Read the model definition and answer for the solid it produces. Units are mm, in the model's axes. Round coordinates to 2 decimals unless told otherwise and drop trailing zeros. Order: outer loops, then holes, each group sorted by start corner. A loop starts at its lowest first (then second) coordinate and runs counter-clockwise, first axis right, second up.
from build123d import *

# Parameters (mm, degrees)
BOSS_EXTRUDE1_DEPTH = 2.54
SKETCH2_R           = 2.159
CUT_EXTRUDE1_DEPTH  = 2.54
FILLET1_R           = 5.08
SKETCH3_W           = 2.54
SKETCH3_H           = 6.35
CUT_EXTRUDE4_DEPTH  = 3.54


with BuildPart() as part:
    # Sketch1 → Boss-Extrude1 (new body)
    with BuildSketch(Plane.XY):
        Polygon((35.56, -47.131), (35.56, 17.131), (-35.56, 17.131), (-35.56, -47.131), (-65.56, -47.131), (-65.56, 47.131), (65.56, 47.131), (65.56, -47.131), align=None)
    extrude(amount=BOSS_EXTRUDE1_DEPTH)

    # Sketch2 → Cut-Extrude1 (cut)
    with BuildSketch(Plane.XY.offset(2.54)):
        with Locations((-56.181, 36.4985)):
            Circle(SKETCH2_R)
        with Locations((-56.181, 26.7195)):
            Circle(SKETCH2_R)
        with Locations((-7.921, 36.4985)):
            Circle(SKETCH2_R)
        with Locations((-7.921, 26.7195)):
            Circle(SKETCH2_R)
        Polygon((-11.477, 41.7055), (-52.625, 41.7055), (-52.625, 21.5125), (-11.477, 21.5125), (-11.477, 31.609), align=None)
    extrude(amount=-CUT_EXTRUDE1_DEPTH, mode=Mode.SUBTRACT)

    # Fillet1
    fillet1_edges = [part.edges().sort_by_distance(p)[0] for p in [
        (-65.56, 47.131, 1.27),
        (65.56, 47.131, 1.27),
        (35.56, -47.131, 1.27),
        (-35.56, -47.131, 1.27),
    ]]
    fillet(fillet1_edges, radius=FILLET1_R)

    # Sketch3 → Cut-Extrude4 (cut, through all)
    with BuildSketch(Plane.XY.offset(2.54)):
        with Locations((-52.625, 31.609)):
            Rectangle(SKETCH3_W, SKETCH3_H)
    extrude(amount=-CUT_EXTRUDE4_DEPTH, mode=Mode.SUBTRACT)


solid = part.part
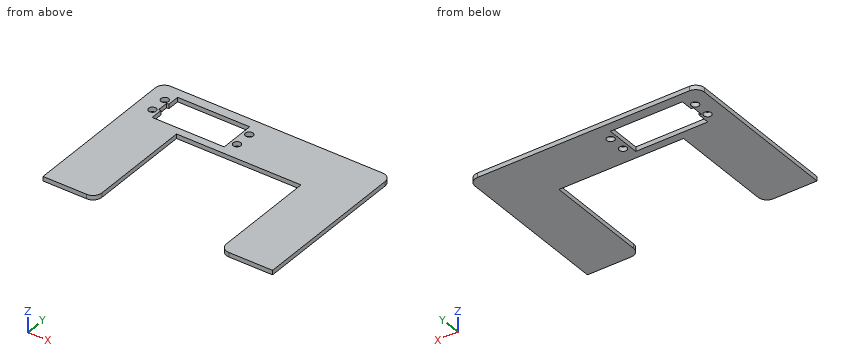
Q1. A cutting plane is placed at D-D, the plane x = 3. Give the vertices of the cut face in (y, z).
Outcome:
outline: (17.13, 0) - (47.13, 0) - (47.13, 2.54) - (17.13, 2.54) - close
Q2. Straight lines are drawn through the part: probe 1 along X at (y, z) = (22, 1.7) (3 decimals); probe 2 along X at (y, z) = (1.5, 0.7); probe 3 along Y at (x, z) = (-46, 0.7). For each, find the intervals that lie inside material, in ascending order.
Outcome:
probe 1: x = -65.56 to -52.625, -11.477 to 65.56
probe 2: x = -65.56 to -35.56, 35.56 to 65.56
probe 3: y = -47.13 to 21.51, 41.71 to 47.13
Q3. A cutting plane is placed at A-A, the plane x = -31. Give the vertices of the cut face in (y, z), plus the area to 3 significant figures.
Outcome:
outline: (17.13, 0) - (21.51, 0) - (21.51, 2.54) - (17.13, 2.54) - close; (41.71, 0) - (47.13, 0) - (47.13, 2.54) - (41.71, 2.54) - close
area: 24.9 mm2
Q4. A cutting plane is placed at C-C, the plane z = 0.8. Give the vertices of the cut face in (x, y) (1 decimal).
Outcome:
outline: (-65.6, -47.1) - (-40.6, -47.1) arc R5.1 ccw to (-35.6, -42.1) - (-35.6, 17.1) - (35.6, 17.1) - (35.6, -42.1) arc R5.1 ccw to (40.6, -47.1) - (65.6, -47.1) - (65.6, 42.1) arc R5.1 ccw to (60.5, 47.1) - (-60.5, 47.1) arc R5.1 ccw to (-65.6, 42.1) - close; hole circle Ø4.3 at (-56.2, 26.7); hole circle Ø4.3 at (-56.2, 36.5); hole (-53.9, 28.4) - (-52.6, 28.4) - (-52.6, 21.5) - (-11.5, 21.5) - (-11.5, 41.7) - (-52.6, 41.7) - (-52.6, 34.8) - (-53.9, 34.8) - close; hole circle Ø4.3 at (-7.9, 26.7); hole circle Ø4.3 at (-7.9, 36.5)
Q5. A cutting plane is placed at B-B, the plane y = 0. Give the vertices of the cut face in (x, z), plus the area to 3 significant figures.
Outcome:
outline: (-65.56, 0) - (-35.56, 0) - (-35.56, 2.54) - (-65.56, 2.54) - close; (35.56, 0) - (65.56, 0) - (65.56, 2.54) - (35.56, 2.54) - close
area: 152 mm2
Q6. Flat-ended cylindrical pins translate along their axes: pin 1 (2.5 mm diameter, centred on x = -7.92, y = 36.5, fed in from -Z); pin 2 (1 mm diameter, centred on x = -29.5, z = 0.5, fed in from -Y). Find the tip coordinate at first contact, or state that the pin passes through.
Outcome:
pin 1: passes through
pin 2: stops at y = 17.13
